Input: dimensioned drawing with shaded views. Units: mm. Origin: part minimum x, y, z. Round coordinates to 2 decimals unless told otherwise and drop trailing zeros. Loops run counter-clockwise (first coordinate to the right, second up) from the corner with the lowest first, then second, coordinate; pieces in that order, holes last. Notation, with made-up numbers: (-15, 25) -> (20, 25) arc R11 cw to (20, 32) -> close; hole circle Ø8 at (51, 63.25). An arc over 180 degrees is marked (long way). Answer as a JSON object with one key per item and string values.
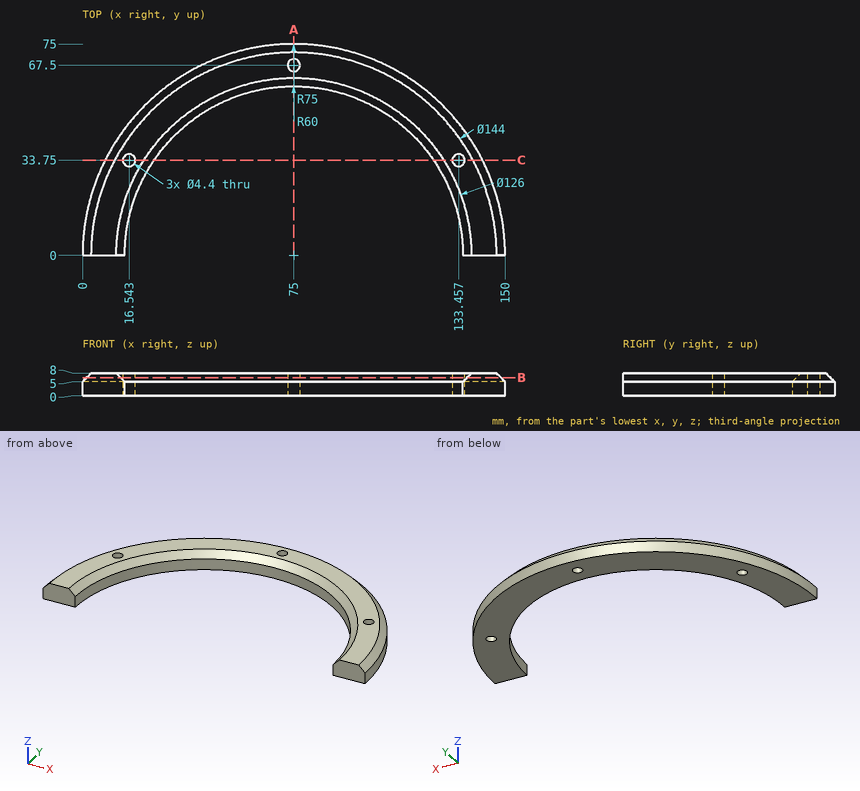
1) Ray query, probe 1 along X at (y, z) = (20.5, 4); probe 2 along X at (y, z) = (13.5, 0.5) (1 decimal); probe 3 along X at (y, z) = (33.5, 6.25) (1 decimal). Return the intervals inside material, ascending.
Output:
{"probe 1": "x = 2.86 to 18.61, 131.39 to 147.14", "probe 2": "x = 1.2 to 16.5, 133.5 to 148.8", "probe 3": "x = 9.3 to 14.4, 18.7 to 23.7, 126.3 to 131.3, 135.6 to 140.7"}
2) Section B-B, the plane z = 6.5. Output: boundary loops of the cut face in (x, y).
Output:
{"outline": "(1.5, 0) -> (13.5, 0) arc R61.5 cw to (136.5, 0) -> (148.5, 0) arc R73.5 ccw to start; hole circle Ø4.4 at (16.54, 33.75); hole circle Ø4.4 at (75, 67.5); hole circle Ø4.4 at (133.46, 33.75)"}
3) Section A-A, the plane x = 75. Output: boundary loops of the cut face in (y, z), plus the area to 3 significant figures.
Output:
{"outline": "(60, 0) -> (65.3, 0) -> (65.3, 8) -> (63, 8) -> (60, 5) -> close; (69.7, 0) -> (75, 0) -> (75, 5) -> (72, 8) -> (69.7, 8) -> close", "area": "75.8 mm^2"}
4) Section C-C, the plane y = 33.75. Count the separate pieces of the cut face and the enclosed holes in it, plus the area to 3 significant figures.
Output:
{"separate pieces": "4", "enclosed holes": "0", "area": "187 mm^2"}
